from build123d import *

# Parameters (mm, degrees)
SKETCH1_R           = 1.778
BOSS_EXTRUDE1_DEPTH = 1.524
BOSS_EXTRUDE2_DEPTH = 1.524


with BuildPart() as part:
    # Sketch1 → Boss-Extrude1 (new body)
    with BuildSketch(Plane.XY):
        with BuildLine():
            ThreePointArc((21.997045256, 12.7), (0, 25.4), (-21.997045256, 12.7))
            ThreePointArc((-21.997045256, 12.7), (-21.997045256, -12.7), (0, -25.4))
            ThreePointArc((0, -25.4), (21.997045256, -12.7), (21.997045256, 12.7))
        make_face()
        with Locations(Location((0, 17.78, 0), (0, 0, 180))):
            Circle(SKETCH1_R, mode=Mode.SUBTRACT)
        with Locations(Location((15.397931679, -8.89, 0), (0, 0, 180))):
            Circle(SKETCH1_R, mode=Mode.SUBTRACT)
        with Locations(Location((-15.397931679, -8.89, 0), (0, 0, 180))):
            Circle(SKETCH1_R, mode=Mode.SUBTRACT)
        with BuildLine():
            Line((-3.81, 17.78), (-3.81, 19.95961673))
            ThreePointArc((-3.81, 19.95961673), (-11.771994053, 16.562685652), (-17.597636205, 10.16))
            ThreePointArc((-17.597636205, 10.16), (-20.229703556, 1.913503077), (-19.190535138, -6.680251576))
            Line((-19.190535138, -6.680251576), (-17.302931679, -5.590443212))
            ThreePointArc((-17.302931679, -5.590443212), (-12.098374891, -6.985), (-13.492931679, -12.189556788))
            Line((-13.492931679, -12.189556788), (-15.380535138, -13.279365153))
            ThreePointArc((-15.380535138, -13.279365153), (-8.457709503, -18.476188729), (0, -20.32))
            ThreePointArc((0, -20.32), (8.457709503, -18.476188729), (15.380535138, -13.279365153))
            Line((15.380535138, -13.279365153), (13.492931679, -12.189556788))
            ThreePointArc((13.492931679, -12.189556788), (12.098374891, -6.985), (17.302931679, -5.590443212))
            Line((17.302931679, -5.590443212), (19.190535138, -6.680251576))
            ThreePointArc((19.190535138, -6.680251576), (20.229703556, 1.913503077), (17.597636205, 10.16))
            ThreePointArc((17.597636205, 10.16), (11.771994053, 16.562685652), (3.81, 19.95961673))
            Line((3.81, 19.95961673), (3.81, 17.78))
            ThreePointArc((3.81, 17.78), (0, 13.97), (-3.81, 17.78))
        make_face(mode=Mode.SUBTRACT)
    extrude(amount=BOSS_EXTRUDE1_DEPTH)

    # Sketch2 → Boss-Extrude2 (add)
    with BuildSketch(Plane.XY.offset(1.524)):
        with BuildLine():
            Line((-3.444175737, 25.165405888), (4.388245609, 23.329352482))
            add(Edge.make_bspline(
                [(-1.351467981, 28.543022953), (2.94701041, 27.179254576), (4.388245609, 23.329352482)],
                knots=[0, 0, 0, 1, 1, 1], degree=2))
            add(Edge.make_bspline(
                [(-1.351467981, 28.543022953), (0.693484877, 25.920519128), (-3.444175737, 25.165405888)],
                knots=[0, 0, 0, 1, 1, 1], degree=2))
        make_face()
        with BuildLine():
            Line((17.527698145, 18.383138953), (20.975648621, 11.114744787))
            add(Edge.make_bspline(
                [(21.473207446, 18.852903941), (23.087027834, 14.641922533), (20.975648621, 11.114744787)],
                knots=[0, 0, 0, 1, 1, 1], degree=2))
            add(Edge.make_bspline(
                [(21.473207446, 18.852903941), (20.697858644, 15.618991025), (17.527698145, 18.383138953)],
                knots=[0, 0, 0, 1, 1, 1], degree=2))
        make_face()
        with BuildLine():
            Line((25.300857823, -2.242006562), (21.767960397, -9.469492432))
            add(Edge.make_bspline(
                [(28.128119692, -5.033836268), (25.84204241, -8.921075819), (21.767960397, -9.469492432)],
                knots=[0, 0, 0, 1, 1, 1], degree=2))
            add(Edge.make_bspline(
                [(28.128119692, -5.033836268), (25.116322693, -6.443955888), (25.300857823, -2.242006562)],
                knots=[0, 0, 0, 1, 1, 1], degree=2))
        make_face()
        with BuildLine():
            Line((14.021955517, -21.178875406), (6.168554008, -22.923008708))
            add(Edge.make_bspline(
                [(13.601984102, -25.129995095), (9.137471969, -25.766322122), (6.168554008, -22.923008708)],
                knots=[0, 0, 0, 1, 1, 1], degree=2))
            add(Edge.make_bspline(
                [(13.601984102, -25.129995095), (10.621683474, -23.654472585), (14.021955517, -21.178875406)],
                knots=[0, 0, 0, 1, 1, 1], degree=2))
        make_face()
        with BuildLine():
            Line((-7.815765289, -24.1676191), (-14.075899364, -19.115031882))
            add(Edge.make_bspline(
                [(-11.166722947, -26.302755058), (-14.447801235, -23.20900233), (-14.075899364, -19.115031882)],
                knots=[0, 0, 0, 1, 1, 1], degree=2))
            add(Edge.make_bspline(
                [(-11.166722947, -26.302755058), (-11.871300044, -23.052688962), (-7.815765289, -24.1676191)],
                knots=[0, 0, 0, 1, 1, 1], degree=2))
        make_face()
        with BuildLine():
            Line((-23.76805542, -8.957652682), (-23.72091342, -0.913046174))
            add(Edge.make_bspline(
                [(-27.526659857, -7.669003983), (-27.153585428, -3.174830406), (-23.72091342, -0.913046174)],
                knots=[0, 0, 0, 1, 1, 1], degree=2))
            add(Edge.make_bspline(
                [(-27.526659857, -7.669003983), (-25.424952498, -5.091760362), (-23.76805542, -8.957652682)],
                knots=[0, 0, 0, 1, 1, 1], degree=2))
        make_face()
        with BuildLine():
            Line((-21.82251504, 12.997608909), (-15.503595851, 17.976481926))
            add(Edge.make_bspline(
                [(-23.158460453, 16.73966351), (-19.412165961, 19.250053568), (-15.503595851, 17.976481926)],
                knots=[0, 0, 0, 1, 1, 1], degree=2))
            add(Edge.make_bspline(
                [(-23.158460453, 16.73966351), (-19.833097147, 16.703367644), (-21.82251504, 12.997608909)],
                knots=[0, 0, 0, 1, 1, 1], degree=2))
        make_face()
    extrude(amount=-BOSS_EXTRUDE2_DEPTH)


solid = part.part
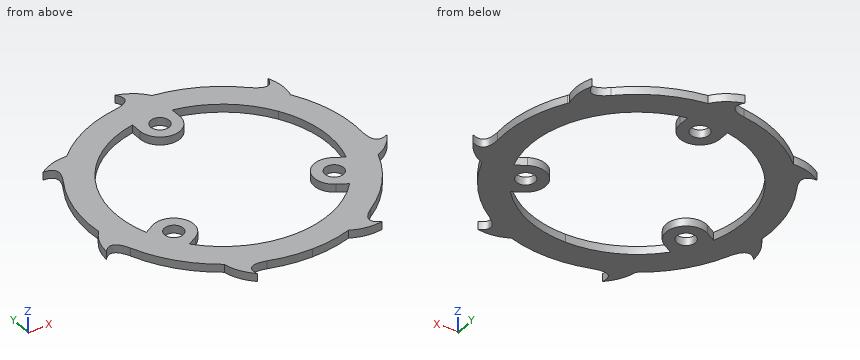
Can you work these out from the model? Positions are in its coordinate system, mm. Give positions to 0.01 mm unless a question says otherwise; leave off trailing zeros. Loops run counter-clockwise (first coordinate to the right, second up) from the corner with the lowest first, then second, coordinate; pieces in that order, holes last. Notation, with made-up numbers: (49, 37.25) -> (107, 37.25) arc R11 cw to (107, 46.25) -> close; hole circle Ø6 at (-9, 12). An arc over 180 degrees is marked (long way). Write item = value, one per line.
1) Will this pin go through, and if not, where does the flat tip stop? pin 1 (0.5 mm diameter, centred on y = 19, z = 0.5, fed in from -X).
Check result:
pin_1 = -17.13
2) Suppose I cut it at B-B on x = 5.5. Write out the boundary of the cut face in (y, z).
Check result:
outline = (-24.8, 0) -> (-19.56, 0) -> (-19.56, 1.52) -> (-24.8, 1.52) -> close; (19.56, 0) -> (24.8, 0) -> (24.8, 1.52) -> (19.56, 1.52) -> close
3) Suppose I cut it at A-A on y = 3. Write out the boundary of the cut face in (x, z).
Check result:
outline = (-25.22, 0) -> (-20.1, 0) -> (-20.1, 1.52) -> (-25.22, 1.52) -> close; (20.1, 0) -> (25.22, 0) -> (25.22, 1.52) -> (20.1, 1.52) -> close
4) I need wall thicknesses on L1, parallel to Y at x = 12, z = 0.8; L2, parallel to Y at x = -15.5, z = 1; L3, parallel to Y at x = 13, z = 0.15. Which ranges of each line are inside material? Lowest first, please. Write a range as from..to.
Check result:
L1 = -25.25..-16.4, -10.61..-7.17, 16.4..22.39
L2 = -20.12..-10.67, -7.11..-5.08, 13.14..20.12
L3 = -25.2..-24.78, -22.04..-15.62, -11.85..-5.93, 15.62..21.82
5) Suppose I cut it at C-C on z = 1.05. Give the number of separate pieces and of enclosed holes in the cut face, then the cut area to 3 significant figures.
Check result:
separate_pieces = 1
enclosed_holes = 4
area = 882 mm2
